Read the model definition and answer for the solid it produces. Units are mm, in the model's axes. Face numbers are marked on the shaded views. Coordinates: 2 decimals unless noted, no trailing zeros. Order: outer loops, then holes, each group sorted by start corner. A loop starts at its lowest first (then second) coordinate and runs counter-clockwise, first axis right, second up.
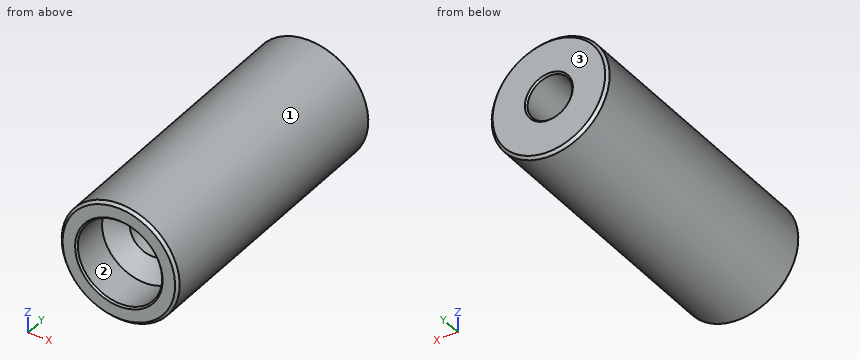
```python
from build123d import *

# Parameters (mm, degrees)
CHAMFER1_SIZE = 0.254
CHAMFER2_SIZE = 0.1524


with BuildPart() as part:
    # Sketch1 → Revolve1 (revolve)
    with BuildSketch(Plane(origin=(0, 0, 0), x_dir=(0, 0, -1), z_dir=(1, 0, 0)), mode=Mode.PRIVATE) as revolve1_sk:
        Polygon((3.9751, 0), (5.5626, 0), (5.5626, 26.9748), (2.1082, 26.9748), (2.1082, 4.67774669), (3.9751, 3.556), align=None)
    revolve(revolve1_sk.sketch.rotate(Axis((0, -4.141094848, 0), (0, -1, 0)), 180), axis=Axis((0, -4.141094848, 0), (0, -1, 0)))

    # Chamfer1
    chamfer1_edges = [part.edges().sort_by_distance(p)[0] for p in [
        (0, 26.9748, -5.5626),
        (0, 0, -5.5626),
    ]]
    chamfer(chamfer1_edges, length=CHAMFER1_SIZE)

    # Chamfer2
    chamfer2_edges = [part.edges().sort_by_distance(p)[0] for p in [
        (0, 26.9748, -2.1082),
        (0, 0, -3.9751),
    ]]
    chamfer(chamfer2_edges, length=CHAMFER2_SIZE)


solid = part.part
```
1) Determine the mould class of the marked faces 1, 2 and 3 for opening direction Z: pulls with the +Z half, pulls with the -Z half, needs draft (parallel to the pull), parting line crosses it, or undercut.
A:
face 1: parting line crosses it
face 2: undercut
face 3: needs draft
2) Flat-ended cylindrical pins translate along their axes: pin 1 Ø4 at (x, z) = (0, 0) entering from +Y; pin 2 Ø2 at (y, z) = (23, -1.5) entering from +X; pin 3 Ø6 at (y, z) = (17.5, 3) entering from +X; pin 4 Ø1.5 at (y, z) = (13, -4.5) entering from +X. Find the tip coordinate at first contact, or state that the pin passes through.
A:
pin 1: passes through
pin 2: stops at x = 5.54
pin 3: stops at x = 5.56
pin 4: stops at x = 4.11
3) Straight lines are drawn through the part: line 1 (X direction, y = 1.5, z = 0); line 2 (X direction, y = 22.25, z = 0); line 3 (Z direction, x = 1.25, y = 8). For each, find the intervals that lie inside material, in ascending order.
A:
line 1: x = -5.56 to -3.98, 3.98 to 5.56
line 2: x = -5.56 to -2.11, 2.11 to 5.56
line 3: z = -5.42 to -1.7, 1.7 to 5.42
4) A cutting plane is placed at B-B, the plane x = 0. Determine the outline of the cut face in (y, z), and give its area (3 significant figures).
A:
outline: (0, -5.31) - (0.25, -5.56) - (26.72, -5.56) - (26.97, -5.31) - (26.97, -2.26) - (26.82, -2.11) - (4.68, -2.11) - (3.56, -3.98) - (0.15, -3.98) - (0, -4.13) - close; (0, 4.13) - (0.15, 3.98) - (3.56, 3.98) - (4.68, 2.11) - (26.82, 2.11) - (26.97, 2.26) - (26.97, 5.31) - (26.72, 5.56) - (0.25, 5.56) - (0, 5.31) - close
area: 171 mm2
5) A cutting plane is placed at C-C, the plane y = 16.75. Determine the outline of the cut face in (x, z), and give its area (3 significant figures).
A:
outline: circle Ø11.13 at (0, 0); hole circle Ø4.22 at (0, 0)
area: 83.2 mm2
6) A cutting plane is placed at A-A, the plane z = 0. Determine the outline of the cut face in (x, y).
A:
outline: (-5.56, 0.25) - (-5.31, 0) - (-4.13, 0) - (-3.98, 0.15) - (-3.98, 3.56) - (-2.11, 4.68) - (-2.11, 26.82) - (-2.26, 26.97) - (-5.31, 26.97) - (-5.56, 26.72) - close; (2.11, 4.68) - (3.98, 3.56) - (3.98, 0.15) - (4.13, 0) - (5.31, 0) - (5.56, 0.25) - (5.56, 26.72) - (5.31, 26.97) - (2.26, 26.97) - (2.11, 26.82) - close
